Check sheet for the modelled part. Datum: model origin and axes. Units: mm. Face numbers are marked on the shaded views. A direction names the side the tool comes from. Give positions to 0.01 mm unless a question says otherwise; leave off trailing zeros. Order: outer loops, then holes, each group sorted by start corner. A loop starts at its lowest first (then second) coordinate and runs counter-clockwise, first axis right, second up. Notation, with made-up numbers: (86.25, -11) - (134.25, -11) arc R22 cw to (134.25, 27) - close; hole circle Ø7 at (-36, -22.75). An arc over 180 degrees is marked (long way). Answer in a Markdown table with one row per item.
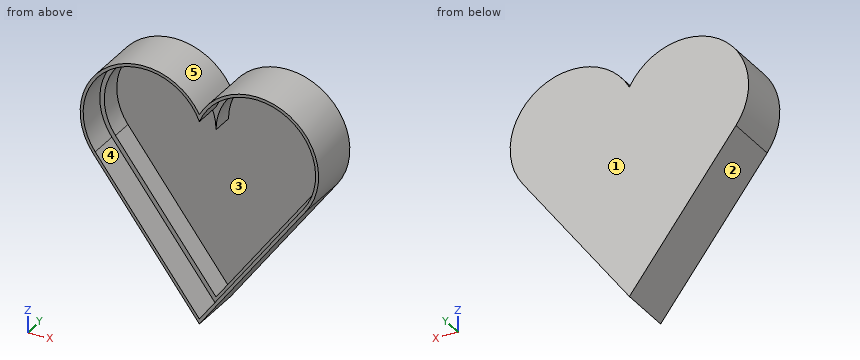
from build123d import *

# Parameters (mm, degrees)
F1_DEPTH = 1
F2_DEPTH = 15
F3_DEPTH = 7


with BuildPart() as f1:
    # F0 (on Front) → F1 (new body)
    with BuildSketch(Plane.XZ):
        with BuildLine():
            ThreePointArc((28.6, -10.2), (24.1268833673, 14.3422452914), (0, 8))
            ThreePointArc((0, 8), (-24.1268833673, 14.3422452914), (-28.6, -10.2))
            Line((-28.6, -10.2), (0, -48.3333333333))
            Line((0, -48.3333333333), (28.6, -10.2))
        make_face()
        with BuildLine():
            ThreePointArc((0, 6.1188234163), (22.9848282263, 14.0954786438), (27.96, -9.72))
            Line((27.96, -9.72), (0, -47))
            Line((0, -47), (-27.96, -9.72))
            ThreePointArc((-27.96, -9.72), (-22.9848282263, 14.0954786438), (0, 6.1188234163))
        make_face(mode=Mode.SUBTRACT)
        with BuildLine():
            Line((0, -47), (27.96, -9.72))
            ThreePointArc((27.96, -9.72), (22.9848282263, 14.0954786438), (0, 6.1188234163))
            ThreePointArc((0, 6.1188234163), (-22.9848282263, 14.0954786438), (-27.96, -9.72))
            Line((-27.96, -9.72), (0, -47))
        make_face()
        with BuildLine():
            ThreePointArc((-27, -9), (-19.7434164903, 14.2302494708), (0, 0))
            ThreePointArc((0, 0), (19.7434164903, 14.2302494708), (27, -9))
            Line((27, -9), (0, -45))
            Line((0, -45), (-27, -9))
        make_face(mode=Mode.SUBTRACT)
        with BuildLine():
            ThreePointArc((27, -9), (19.7434164903, 14.2302494708), (0, 0))
            ThreePointArc((0, 0), (-19.7434164903, 14.2302494708), (-27, -9))
            Line((-27, -9), (0, -45))
            Line((0, -45), (27, -9))
        make_face()
    extrude(amount=F1_DEPTH)

    # F0 (on Front) → F2 (join)
    with BuildSketch(Plane.XZ):
        with BuildLine():
            ThreePointArc((28.6, -10.2), (24.1268833673, 14.3422452914), (0, 8))
            ThreePointArc((0, 8), (-24.1268833673, 14.3422452914), (-28.6, -10.2))
            Line((-28.6, -10.2), (0, -48.3333333333))
            Line((0, -48.3333333333), (28.6, -10.2))
        make_face()
        with BuildLine():
            ThreePointArc((0, 6.1188234163), (22.9848282263, 14.0954786438), (27.96, -9.72))
            Line((27.96, -9.72), (0, -47))
            Line((0, -47), (-27.96, -9.72))
            ThreePointArc((-27.96, -9.72), (-22.9848282263, 14.0954786438), (0, 6.1188234163))
        make_face(mode=Mode.SUBTRACT)
    extrude(amount=F2_DEPTH)

    # F0 (on Front) → F3 (join)
    with BuildSketch(Plane.XZ):
        with BuildLine():
            Line((0, -47), (27.96, -9.72))
            ThreePointArc((27.96, -9.72), (22.9848282263, 14.0954786438), (0, 6.1188234163))
            ThreePointArc((0, 6.1188234163), (-22.9848282263, 14.0954786438), (-27.96, -9.72))
            Line((-27.96, -9.72), (0, -47))
        make_face()
        with BuildLine():
            ThreePointArc((-27, -9), (-19.7434164903, 14.2302494708), (0, 0))
            ThreePointArc((0, 0), (19.7434164903, 14.2302494708), (27, -9))
            Line((27, -9), (0, -45))
            Line((0, -45), (-27, -9))
        make_face(mode=Mode.SUBTRACT)
    extrude(amount=F3_DEPTH)


solid = f1.part
(1) Cross-section at B-B, the plane y = -8. Record the cut outline in (x, z).
Geometry says:
| item | result |
|---|---|
| outline | (-28.6, -10.2) - (0, -48.33) - (28.6, -10.2) arc R17 ccw (long way) to (0, 8) arc R17 ccw (long way) to start; hole (-27.96, -9.72) - (0, -47) - (27.96, -9.72) arc R16.2 ccw (long way) to (0, 6.12) arc R16.2 ccw (long way) to start |
(2) Cross-section at D-D, the plane z = 7. Record the cut outline in (x, y), then the cut area to 3 significant figures.
Geometry says:
| item | result |
|---|---|
| outline | (-30.49, -15) - (-29.61, -15) - (-29.61, -7) - (-28.27, -7) - (-28.27, -1) - (-1.73, -1) - (-1.73, -7) - (-0.39, -7) - (-0.39, -15) - (0.39, -15) - (0.39, -7) - (1.73, -7) - (1.73, -1) - (28.27, -1) - (28.27, -7) - (29.61, -7) - (29.61, -15) - (30.49, -15) - (30.49, 0) - (-30.49, 0) - close |
| area | 129 mm² |
(3) Cross-section at C-C, the plane x = -10. Record the cut outline in (y, z), then the cut area to 3 significant figures.
Geometry says:
| item | result |
|---|---|
| outline | (-15, -35) - (0, -35) - (0, 16.25) - (-15, 16.25) - (-15, 15.41) - (-7, 15.41) - (-7, 14.14) - (-1, 14.14) - (-1, -31.67) - (-7, -31.67) - (-7, -33.67) - (-15, -33.67) - close |
| area | 101 mm² |
(4) Gauge pin test, flat ends, axial feed: P1, Ø1.5, axis at x = 13.5, y = -10, coming from the +Z side; P2, Ø2, axis at y = -10.5, z = -38, coming from the +X side; P3, Ø18, axis at x = -2, z = -14.5, coming from the -Y side. Record the tip position at first contact, or that the pin passes through.
Geometry says:
| item | result |
|---|---|
| P1 | z = 16.98 |
| P2 | x = 8.5 |
| P3 | y = -1 |
(5) Cross-section at A-A, the plane z = -36. Record the cut outline in (x, y), then the cut area to 3 significant figures.
Geometry says:
| item | result |
|---|---|
| outline | (-9.25, -15) - (-8.25, -15) - (-8.25, -7) - (-6.75, -7) - (-6.75, -1) - (6.75, -1) - (6.75, -7) - (8.25, -7) - (8.25, -15) - (9.25, -15) - (9.25, 0) - (-9.25, 0) - close |
| area | 64.5 mm² |
(6) Thickness scan on L1, parallel to X at y = -12.75, z = 0; L2, parallel to Y at x = 21, z = 0; L3, parallel to Z at x = 7.5, y = -13.75. Record the ranges inside material, lowest first.
Geometry says:
| item | result |
|---|---|
| L1 | -32 to -31.2, 31.2 to 32 |
| L2 | -1 to 0 |
| L3 | -38.33 to -37, 14.36 to 15.26 |
(7) Mould release check, pull along Z, two halves, no side actions. Record for the marked faces 1, 2 and 3: pulls with the +Z half, pulls with the -Z half, needs draft (parallel to the pull), parting line crosses it, or undercut.
Geometry says:
| item | result |
|---|---|
| face 1 | needs draft |
| face 2 | pulls with the -Z half |
| face 3 | undercut |
(8) Access from +Z, -Z, +X, -X, +Y, -Y to the whole of each face (thin tool, end or side, straight path). Record for the marked faces 4 and 5.
Geometry says:
| item | result |
|---|---|
| face 4 | -Y |
| face 5 | +Y, -Y |
